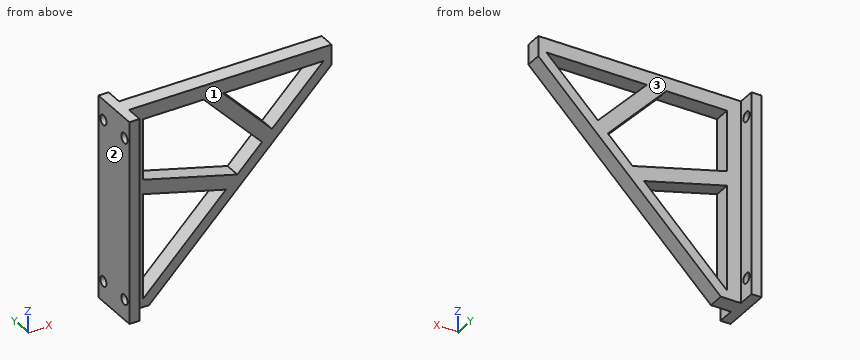
```python
from build123d import *

# Parameters (mm, degrees)
PAD_DEPTH    = 8
SKETCH001_W  = 100
SKETCH001_H  = 25
SKETCH001_R  = 2.5
PAD001_DEPTH = 5


with BuildPart() as part:
    # Sketch → Pad (new body)
    with BuildSketch(Plane.XZ):
        Polygon((0, 0), (0, 100), (100, 100), (100, 90.074147), (9.925853, 0), align=None)
        Polygon((6.854785, 93.145215), (36.854785, 93.145215), (65.676567, 62.821781), (53.501145, 50.64636), (6.854785, 63.145215), align=None, mode=Mode.SUBTRACT)
        Polygon((47.852116, 44.997331), (6.854785, 55.982532), (6.854785, 4), align=None, mode=Mode.SUBTRACT)
        Polygon((70.570346, 67.715561), (46.399999, 93.145215), (96, 93.145215), align=None, mode=Mode.SUBTRACT)
    extrude(amount=PAD_DEPTH)

    # Sketch001 (on DatumPlane) → Pad001 (join)
    with BuildSketch(Plane(origin=(0, 0, 0), x_dir=(0, 0, -1), z_dir=(-1, 0, 0))):
        with Locations((-50, 4)):
            Rectangle(SKETCH001_W, SKETCH001_H)
        with Locations((-90, 12.5)):
            Circle(SKETCH001_R, mode=Mode.SUBTRACT)
        with Locations((-10, 12.5)):
            Circle(SKETCH001_R, mode=Mode.SUBTRACT)
        with Locations((-90, -4.5)):
            Circle(SKETCH001_R, mode=Mode.SUBTRACT)
        with Locations((-10, -4.5)):
            Circle(SKETCH001_R, mode=Mode.SUBTRACT)
    extrude(amount=PAD001_DEPTH)


solid = part.part
```
Verification items for the finished model (mm, model axes). Face numbers are marked on the shaded views. A direction names the side the tool comes from. Give positions to 0.01 mm unless a question says otherwise; leave off trailing zeros. Order: outer loops, then holes, each group sorted by start corner. A loop starts at its lowest first (then second) coordinate and runs counter-clockwise, first axis right, second up. Notation, with made-up numbers: M 3,-32.75 L 55,-32.75 A15 cw 55,-14.75 Z; hole C 41.25,-32 d10. An arc over 180 degrees is marked long. Answer in a Markdown table with one row per item. Add a question column.
Item 1: Scan lines: probe 1 along Y at (x, z) = (-2.75, 90); probe 2 along Z at (x, y) = (-3.6, 4.5); probe 3 along Z at (x, y) = (44, -1). Record each from-to range of solid material in increasing order. Write a range as from..to.
Item 2: Section check A-A, the plane y = 4.5. Enter the section's corners in (x, z).
Item 3: Gauge pin test, flat ends, axial feed: pin 1 (6.5 mm diameter, centred on y = 4.5, z = 10, fed in from +X); pin 2 (4 mm diameter, centred on x = 15, y = -4, fed in from -Z); pin 3 (6.5 mm diameter, centred on x = 76.5, y = -5, fed in from -Z); pin 4 (6 mm diameter, centred on y = 4.5, z = 90, fed in from -X). Record the tip position at first contact, or that the pin passes through.
Item 4: Section check B-B, the plane x = 35. Enter the section's corners in (y, z).
Item 5: Section check D-D, the plane x = 85. Enter the section's corners in (y, z).
Item 6: Tool access check on the marked faces 1, 2 and 3. Record the directions out of +Z, -Z, +X, -X, +Y, -Y that give a thin tool (end or side, any length) a straight path to the whole face; none if there is none.
Item 7: Section check C-C, the plane z = 16. Enter the section's corners in (x, y), and give its area (3 significant figures).
Filled sheet:
| question | item | result |
|---|---|---|
| 1 | probe 1 | y = -16.5..-15, -10..2, 7..8.5 |
| 1 | probe 2 | z = 0..7.5, 12.5..87.5, 92.5..100 |
| 1 | probe 3 | z = 34.07..41.15, 46.03..53.19, 85.63..100 |
| 2 | outline | M -5,0 L 0,0 L 0,7.5 L -5,7.5 Z; M -5,12.5 L 0,12.5 L 0,87.5 L -5,87.5 Z; M -5,92.5 L 0,92.5 L 0,100 L -5,100 Z |
| 3 | pin 1 | stops at x = 0 |
| 3 | pin 2 | stops at z = 3.07 |
| 3 | pin 3 | stops at z = 63.32 |
| 3 | pin 4 | stops at x = -5 |
| 4 | outline | M -8,25.07 L 0,25.07 L 0,32.15 L -8,32.15 Z; M -8,48.44 L 0,48.44 L 0,55.6 L -8,55.6 Z; M -8,93.15 L 0,93.15 L 0,100 L -8,100 Z |
| 5 | outline | M -8,75.07 L 0,75.07 L 0,82.15 L -8,82.15 Z; M -8,93.15 L 0,93.15 L 0,100 L -8,100 Z |
| 6 | face 1 | +Z, -Z, +X, -Y |
| 6 | face 2 | +Z, -Z, -X, +Y, -Y |
| 6 | face 3 | +Z, -Z, +X, +Y |
| 7 | outline | M -5,-16.5 L 0,-16.5 L 0,-8 L 6.85,-8 L 6.85,0 L 0,0 L 0,8.5 L -5,8.5 Z; M 18.85,-8 L 25.93,-8 L 25.93,0 L 18.85,0 Z |
| 7 | area | 236 mm^2 |
